CAD build for the part. Positions are in the model's coordinates, mm. Face numbers are marked on the shaded views. A direction names the side the tool comes from. Coordinates: 2 decimals unless noted, no trailing zeros. Loops run counter-clockwise (first coordinate to the right, second up) from the corner with the lowest first, then second, coordinate; pieces in that order, holes last. Notation, with made-up numbers: (-5, 82.5) -> (40, 82.5) arc R7 ccw to (40, 87.5) -> close; hole circle Ø4 at (35, 20.5). An arc over 180 degrees is marked (long way). Answer as CSV lines item,"result". Start each with the question number.
from build123d import *

# Parameters (mm, degrees)
F3_D     = 19.05
F3_DEPTH = 25.4
F4_D     = 19.05
F4_DEPTH = 25.4
F6_DEPTH = 3.175
F7_R     = 1.27


with BuildPart() as f2:
    # F0 (on Front) → F2 (revolve)
    with BuildSketch(Plane.XZ):
        with BuildLine():
            ThreePointArc((2.54, 13.73715), (1.275325, 13.911666), (0, 13.97))
            Line((0, 13.97), (0, -13.97))
            ThreePointArc((0, -13.97), (13.911666, -1.275325), (2.54, 13.73715))
        make_face()
        with BuildLine():
            Line((0, 17.78), (0, 13.97))
            ThreePointArc((0, 13.97), (1.275325, 13.911666), (2.54, 13.73715))
            Line((2.54, 13.73715), (2.54, 17.78))
            Line((2.54, 17.78), (0, 17.78))
        make_face()
    revolve(axis=Axis((0, 0, 6.35), (0, 0, 1)))

    # F3
    with Locations(Plane.XZ):
        with Locations((0, 0)):
            Hole(F3_D / 2, depth=F3_DEPTH)

    # F4
    with Locations(Plane(origin=(0, 0, 0), x_dir=(1, 0, 0), z_dir=(0, 1, 0))):
        with Locations((0, 0)):
            Hole(F4_D / 2, depth=F4_DEPTH)

    # F5 (on Right) → F6 (join, symmetric)
    with BuildSketch(Plane.YZ):
        Polygon((0, 28.143921), (0, 17.78), (25.4, 17.78), (23.45404, 22.472509), align=None)
        Polygon((-25.4, 17.78), (0, 17.78), (0, 28.143921), (-23.45404, 22.472509), align=None)
    extrude(amount=F6_DEPTH, both=True)

    # F7
    f7_edges = [f2.edges().sort_by_distance(p)[0] for p in [
        (3.175, -11.72702, 25.308215),
        (-3.175, -11.72702, 25.308215),
        (3.175, 11.72702, 25.308215),
        (-3.175, 11.72702, 25.308215),
        (3.175, 24.42702, 20.126254),
        (3.175, -24.42702, 20.126254),
        (-3.175, -24.42702, 20.126254),
        (-3.175, 24.42702, 20.126254),
    ]]
    fillet(f7_edges, radius=F7_R)


solid = f2.part
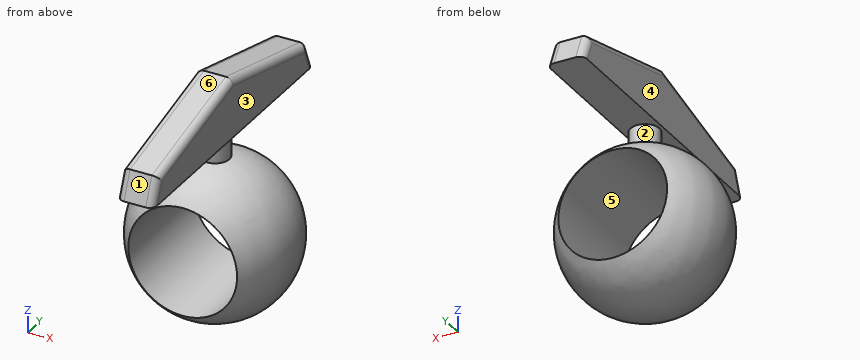
Item 1: Saw through at A-A (y = -6.5). Count the separate pieces of the cut face and the enclosed holes in it, plus the area to 3 significant figures.
Item 2: Wall check: probe 1 along Z at (x, y) = (3, 6.5); probe 2 along X at (y, z) = (-4, 0) (3 decimals); probe 3 along X at (y, z) = (4.75, 0) (3 decimals). Give the ranges that are in metal, low to high.
Item 3: Saw through at B-B (z = 15.5). Write the cut outline in (x, y), plus the area to 3 significant figures.
Item 4: Which spindle directions (+Z, -Z, +X, -X, +Y, -Y) get a long thin tool onto all of the face, cutting with end or side? Do the marked faces 1, 2 and 3. Say none if no direction does.
Item 5: Flat gauge pins, fed straight in: pin 1 Ø5 at (x, z) = (-6.5, -8.5) entering from +Y; pin 2 Ø10 at (x, z) = (3, 3.5) entering from -Y; pin 3 Ø10 at (x, z) = (-1.5, 2.5) entering from +Y; pin 4 Ø12 at (y, z) = (-6, -4.5) entering from +X. Where does each tip first touch, or does it go through?
Item 6: Two-plate mould, pull along Z, no slides. Class the marked faces 4, 5 and 6: pulls with the +Z half, pulls with the -Z half, needs draft (parallel to the pull), parting line crosses it, or undercut.
Geometry check:
1,separate pieces,"2"
1,enclosed holes,"1"
1,area,"250 mm2"
2,probe 1,"-12 to -9.04, 9.04 to 12, 17.78 to 25.93"
2,probe 2,"-13.385 to -9.525, 9.525 to 13.385"
2,probe 3,"-13.138 to -9.525, 9.525 to 13.138"
3,outline,"circle Ø5.08 at (0, 0)"
3,area,"20.3 mm2"
4,face 1,"+Z, +X, -X, -Y"
4,face 2,"none"
4,face 3,"+Z, +X, +Y, -Y"
5,pin 1,"y = 10.22"
5,pin 2,"y = -10.22"
5,pin 3,"through"
5,pin 4,"x = 13.89"
6,face 4,"needs draft"
6,face 5,"undercut"
6,face 6,"pulls with the +Z half"
